Solid Edge part; units mm, degrees
sketch "Sketch1" plane through (0, 0, 0) normal (0, -1, 0) x (1, 0, 0)
  line L0 (9.5, 16.5) -> (9.5, -16.5)
  line L1 (13.5, -16.5) -> (9.5, -16.5)
  line L2 (13.5, -21.5) -> (13.5, -16.5)
  line L3 (22, -21.5) -> (13.5, -21.5)
  line L4 (22, -21.5) -> (22, -1.5)
  line L5 (22, -1.5) -> (38.435, -1.5)
  line L6 (38.435, -1.5) -> (38.435, 6.5)
  line L7 (38.435, 6.5) -> (15.5, 6.5)
  line L8 (15.5, 6.5) -> (15.5, 21.5)
  line L9 (15.5, 21.5) -> (13.5, 21.5)
  line L10 (13.5, 21.5) -> (13.5, 16.5)
  line L11 (13.5, 16.5) -> (9.5, 16.5)
  dimension "D1" = 38.435
  dimension "D2" = 15.5
  dimension "D3" = 13.5
  dimension "D4" = 13.5
revolve "RevolvedProtrusion1" add sketch "Sketch1" angle 360 about axis through (0, 0, 0) along (0, 0, 1)
hole "Hole1" at (0, 32.5, 6.5) direction (0, 0, -1) diameter 6.5 end up to next
pattern_circular "Pattern1" count 6 over 360 about axis through (0, 0, 6.5) along (0, 0, -1) of "Hole1"
Here's how the part is built. I have some questions about the finished solid (model axes, mm). A direction names the side the tool comes from. Give positions to 0.01 mm unless a question says otherwise; leave off trailing zeros. Loops run counter-clockwise (first coordinate to the right, second up) from the corner with the lowest first, then second, coordinate; pieces in that order, holes last. Notation, with made-up numbers: (-26.75, 56.5) -> (4.25, 56.5) arc R36 cw to (4.25, 91.5) -> close; hole circle Ø11 at (0.25, 31.25). An arc over 180 degrees is marked (long way). One line per item, written item: value.
Q1. We'd pull the mould along Y, two halves only. Please class faces 4 (the face through (-3.2, 9.2, -16.5)), 5 (the face through (-5, 13, 21.5)), 6 (the face through (-4.769, -21.477, -11.36)): pulls with the +Y half, pulls with the -Y half, needs draft (parallel to the pull), parting line crosses it, or undercut.
Answers follow:
face 4: undercut
face 5: needs draft
face 6: parting line crosses it
Q2. If I drill on line 1 along Y through (x, z) = (0, 5) (3 decimals); line 2 along Y through (x, z) = (0, 20); line 3 along Z through (x, y) = (5.5, -34), over which ranges is the centre line in solid material (lowest first)?
Answers follow:
line 1: -38.435 to -35.75, -29.25 to -9.5, 9.5 to 29.25, 35.75 to 38.435
line 2: -15.5 to -13.5, 13.5 to 15.5
line 3: -1.5 to 6.5
Q3. Suppose I cut it at C-C on z = 10.5. Please give me the cut outline in (x, y), then the cut area to 3 significant figures.
Answers follow:
outline: circle Ø31 at (0, 0); hole circle Ø19 at (0, 0)
area: 471 mm^2
Q4. On a 3-axis mill with a long thin cutter (end or side, diameter ignored), from which of +Z, -Z, +X, -X, +Y, -Y can I reach the whole of each face in a straight line? I mean faces 1 (the face through (17, 1, 6.5)), 2 (the face through (36.66, 11.54, 2.56)), 3 (the face through (17, -17, -1.5)). Say none if no direction works.
Answers follow:
face 1: +Z
face 2: +Z, -Z
face 3: -Z
Q5. Suppose I cut it at B-B on x = 0. State how many separate pieces and enclosed holes the cut face has, then the cut area to 3 significant figures.
Answers follow:
separate pieces: 4
enclosed holes: 0
area: 959 mm^2
Q6. Suppose I cut it at A-A on y = 0. Please give me the cut outline in (x, z) (3 decimals).
Answers follow:
outline: (-38.435, -1.5) -> (-22, -1.5) -> (-22, -21.5) -> (-13.5, -21.5) -> (-13.5, -16.5) -> (-9.5, -16.5) -> (-9.5, 16.5) -> (-13.5, 16.5) -> (-13.5, 21.5) -> (-15.5, 21.5) -> (-15.5, 6.5) -> (-38.435, 6.5) -> close; (9.5, -16.5) -> (13.5, -16.5) -> (13.5, -21.5) -> (22, -21.5) -> (22, -1.5) -> (38.435, -1.5) -> (38.435, 6.5) -> (15.5, 6.5) -> (15.5, 21.5) -> (13.5, 21.5) -> (13.5, 16.5) -> (9.5, 16.5) -> close
Q7. I'm going to push flat-ended pins straight in: pin 1 Ø8.5 at (x, y) = (-28.15, 16.25) entering from -Z; pin 2 Ø8 at (y, z) = (-4, 0.5) entering from -X (3 decimals); pin 3 Ø10 at (x, y) = (21, -4.5) entering from +Z; pin 4 Ø6 at (x, y) = (28.15, -16.25) entering from +Z. Where does each tip first touch, or does it pass through?
Answers follow:
pin 1: z = -1.5
pin 2: x = -38.435
pin 3: z = 6.5
pin 4: through
Q8. Suppose I cut it at D-D on y = -11.5. Please give me the cut outline in (x, z) (3 decimals).
Answers follow:
outline: (-36.674, -1.5) -> (-18.755, -1.5) -> (-18.755, -21.5) -> (-7.071, -21.5) -> (-7.071, -16.5) -> (7.071, -16.5) -> (7.071, -21.5) -> (18.755, -21.5) -> (18.755, -1.5) -> (36.674, -1.5) -> (36.674, 6.5) -> (10.392, 6.5) -> (10.392, 21.5) -> (7.071, 21.5) -> (7.071, 16.5) -> (-7.071, 16.5) -> (-7.071, 21.5) -> (-10.392, 21.5) -> (-10.392, 6.5) -> (-36.674, 6.5) -> close
